from build123d import *

# Parameters (mm, degrees)
F0_R     = 100.75
F1_DEPTH = 4
F2_DEPTH = 4
F3_DEPTH = 8
F0_R_2   = 105.75
F4_DEPTH = 7
F6_R     = 1
F7_R     = 1
F8_D     = 6.7564
F9_R     = 1


with BuildPart() as f1:
    # F0 (on Front) → F1 (new body)
    with BuildSketch(Plane.XZ):
        Circle(F0_R)
        Polygon((80.5, 46.4766966698), (80.5, -46.4766966698), (0, -92.9533933395), (-80.5, -46.4766966698), (-80.5, 46.4766966698), (0, 92.9533933395), align=None, mode=Mode.SUBTRACT)
    extrude(amount=F1_DEPTH)

    # F0 (on Front) → F4 (join)
    with BuildSketch(Plane.XZ):
        Circle(F0_R_2)
        Circle(F0_R, mode=Mode.SUBTRACT)
    extrude(amount=F4_DEPTH)


with BuildPart() as f1b:
    # F0 (on Front) → F1, piece 2 (new body)
    with BuildSketch(Plane.XZ):
        Polygon((77.5, -44.7446458622), (77.5, 44.7446458622), (0, 89.4892917244), (-77.5, 44.7446458622), (-77.5, -44.7446458622), (0, -89.4892917244), align=None)
        Polygon((39.5, 22.805335633), (39.5, -22.805335633), (0, -45.610671266), (-39.5, -22.805335633), (-39.5, 22.805335633), (0, 45.610671266), align=None, mode=Mode.SUBTRACT)
    extrude(amount=F1_DEPTH)

    # F0 (on Front) → F3 (join)
    with BuildSketch(Plane.XZ):
        Polygon((0, -45.610671266), (39.5, -22.805335633), (39.5, 22.805335633), (0, 45.610671266), (-39.5, 22.805335633), (-39.5, -22.805335633), align=None)
        Polygon((34.5, 19.918584287), (34.5, -19.918584287), (0, -39.8371685741), (-34.5, -19.918584287), (-34.5, 19.918584287), (0, 39.8371685741), align=None, mode=Mode.SUBTRACT)
    extrude(amount=F3_DEPTH)


with BuildPart() as f2:
    # F0 (on Front) → F2 (new body)
    with BuildSketch(Plane.XZ):
        Polygon((0, -92.9533933395), (80.5, -46.4766966698), (80.5, 46.4766966698), (0, 92.9533933395), (-80.5, 46.4766966698), (-80.5, -46.4766966698), align=None)
        Polygon((0, 89.4892917244), (77.5, 44.7446458622), (77.5, -44.7446458622), (0, -89.4892917244), (-77.5, -44.7446458622), (-77.5, 44.7446458622), align=None, mode=Mode.SUBTRACT)
    extrude(amount=F2_DEPTH)


with BuildPart() as f1_1:
    add(f1.part)

    # F5: union F1b, F2
    add(f1b.part)
    add(f2.part)

    # F6
    f6_edges = [f1_1.edges().sort_by_distance(p)[0] for p in [
        (19.75, -8, 34.208003),
        (39.5, -8, 0),
        (19.75, -8, -34.208003),
        (-19.75, -8, -34.208003),
        (-39.5, -8, 0),
        (-19.75, -8, 34.208003),
    ]]
    fillet(f6_edges, radius=F6_R)

    # F7
    f7_edges = [f1_1.edges().sort_by_distance(p)[0] for p in [
        (-100.75, -4, 0),
        (-105.75, 0, 0),
        (-17.25, 0, 29.877876),
        (17.25, 0, 29.877876),
        (34.5, 0, 0),
        (17.25, 0, -29.877876),
        (-17.25, 0, -29.877876),
        (-34.5, 0, 0),
    ]]
    fillet(f7_edges, radius=F7_R)

    # F8 (through all)
    with Locations(Plane(origin=(0, 0, 0), x_dir=(1, 0, 0), z_dir=(0, 1, 0))):
        with Locations((-46.125, -79.8908434991), (46.125, -79.8908434991), (92.25, 0), (46.125, 79.8908434991), (-46.125, 79.8908434991), (-92.25, 0)):
            Hole(F8_D / 2)

    # F9
    f9_edges = [f1_1.edges().sort_by_distance(p)[0] for p in [
        (-100.75, -7, 0),
    ]]
    fillet(f9_edges, radius=F9_R)


solid = f1_1.part
Design review of the part built by this model. Coordinates are the model's own, in mm. A direction names the side the tool comes from. Give positions to 0.01 mm unless a question says otherwise; leave off trailing zeros. Order: outer loops, then holes, each group sorted by start corner. A loop starts at its lowest first (then second) coordinate and runs counter-clockwise, first axis right, second up.
1. For pin 1 Ø11 at (x, z) = (46.12, -79.89) entering from +Y; pin 2 Ø2.5 at (y, z) = (-5, -9.5) entering from -X; pin 3 Ø5.5 at (x, z) = (92.25, 0) entering from -Y; pin 4 Ø11 at (x, z) = (-46.12, 79.89) entering from -Y, all flat-tipped, find the tip position at first contact; note any pin that passes through.
Solution:
pin 1: stops at y = 0
pin 2: stops at x = -105.43
pin 3: passes through
pin 4: stops at y = -4
2. Add section A-A, the plane z = 0. State how many separate pieces and enclosed holes the cut face has, then the cut area to 3 significant figures.
Solution:
separate pieces: 4
enclosed holes: 0
area: 585 mm2
3. To check wall thickness, follow L1, parallel to Z at x = 0, y = -5.75; L2, parallel to Z at x = 17, y = -5; L3, parallel to Y at x = 4, z = 44. State the ranges of each line that lie inside material, in increasing order.
Solution:
L1: z = -105.75 to -100.75, -45.61 to -39.84, 39.84 to 45.61, 100.75 to 105.75
L2: z = -104.37 to -99.31, -35.8 to -30.02, 30.02 to 35.8, 99.31 to 104.37
L3: y = -4 to 0
4. Add section B-B, the plane y = -2.75. State the section outline as (x, z) points (3 decimals).
Solution:
outline: circle Ø211.5 at (0, 0); hole circle Ø6.756 at (-92.25, 0); hole circle Ø6.756 at (-46.125, -79.891); hole circle Ø6.756 at (-46.125, 79.891); hole (-34.5, -19.919) - (0, -39.837) - (34.5, -19.919) - (34.5, 19.919) - (0, 39.837) - (-34.5, 19.919) - close; hole circle Ø6.756 at (46.125, -79.891); hole circle Ø6.756 at (46.125, 79.891); hole circle Ø6.756 at (92.25, 0)
5. Mouldability with a two-part tool opening along Z and no side actions: class faces 5 (the cylindrical face through (19.323, -7.715, 34.107)), 6 (the cylindrical face through (48.615, -2.028, -82.174)), 7 (the flat face through (45, 0, 1)) as +Z half, -Z half, draft (parallel to the pull), parting line (faces both ways), or undercut.
Solution:
face 5: +Z half
face 6: undercut
face 7: draft
6. Tool access review of faces 1 (the flat face through (17.49, -4.45, -29.74)), 2 (the cylindrical face through (-17.14, -0.3, 30.27)), 3 (the flat face through (-20.026, -5.479, -34.048)), 4 (the flat face through (-14, -8, -33)): name each direction out of +Z, -Z, +X, -X, +Y, -Y from which nothing blocks a thin tool from reaching the whole face with its end or side.
Solution:
face 1: +Y, -Y
face 2: +Y
face 3: -Y
face 4: +Z, -Z, +X, -X, -Y
